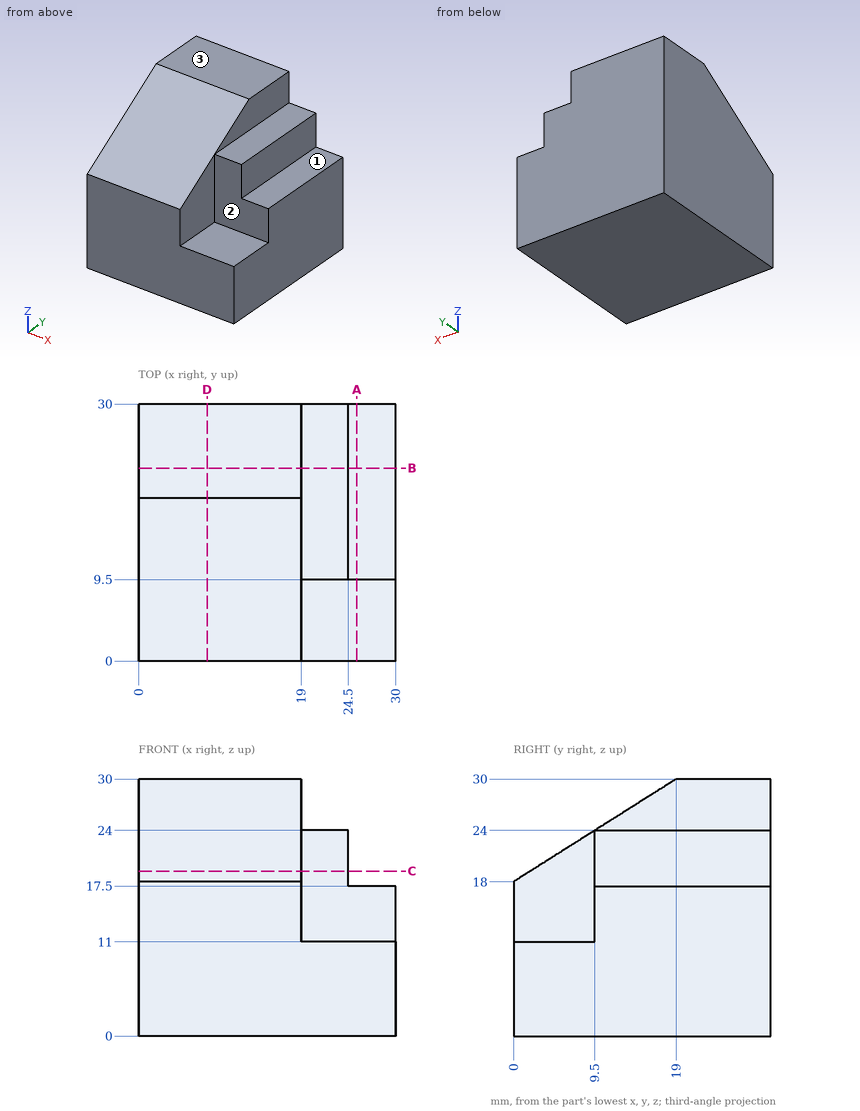
Drawing for the job (mm, zero at the part's lowest x, y, z). A direction names the side the tool comes from. Give positions to 0.01 mm unless a question says otherwise; leave off trailing zeros. Write each loop counter-clockwise with the first axis right and the second up, starting at its lowest first coordinate (ties: lowest second). Pieces come first, ordered by that corner, then holes. Notation, with made-up numbers: M 82,-23 L 93,-23 A22 ccw 93,-7 Z; hole C 37.25,-20.75 d1. An arc over 180 degrees is marked long. Return JSON: item names as keys, results as strings. Group by question number.
(1) Band-saw the part on C-C (z = 19.25). Give the cut face in (x, y), and give its area (3 significant figures).
(2) Flat gauge pins, fed straight in: pin 1 Ø1.5 at (x, y) = (21, 11.5) entering from -Z; pin 2 Ø1.6 at (x, y) = (22, 23.5) entering from +Z; pin 3 Ø5 at (y, z) = (19.5, 28) entering from +X; pin 4 Ø3 at (y, z) = (21, 20) entering from +X. Where does each tip first touch, or does it go through?
(3) Band-saw the part on B-B (y = 22.5). Give the cut face in (x, z).
(4) 3-axis set-ups, long thin cutter, end or side, ignore diameter. For the marked faces 1, 2 and 3: which of +Z, -Z, +X, -X, +Y, -Y reach the whole face in a straight line?
(5) Band-saw the part on D-D (x = 8). Give the cut face in (y, z).
(6) Drill centre lines: L1, parallel to Y at x = 20.5, z = 12; L2, parallel to X at y = 5.75, z = 15.5; L3, parallel to X at y = 25, z = 20.5. Where is each one in solid material? Low to high. Write a range as [from, to].
(7) Band-saw the part on A-A (x = 25.5). Give the cut face in (y, z), and give its area (3 significant figures).
Entries:
{
 "1": {"outline": "M 0,1.98 L 19,1.98 L 19,9.5 L 24.5,9.5 L 24.5,30 L 0,30 Z", "area": "645 mm^2"},
 "2": {"pin 1": "stops at z = 0", "pin 2": "stops at z = 24", "pin 3": "stops at x = 19", "pin 4": "stops at x = 24.5"},
 "3": {"outline": "M 0,0 L 30,0 L 30,17.5 L 24.5,17.5 L 24.5,24 L 19,24 L 19,30 L 0,30 Z"},
 "4": {"face 1": "+Z, +X, +Y, -Y", "face 2": "+Z, +X, -Y", "face 3": "+Z, +X, -X, +Y, -Y"},
 "5": {"outline": "M 0,0 L 30,0 L 30,30 L 19,30 L 0,18 Z"},
 "6": {"L1": "y = [9.5, 30]", "L2": "x = [0, 19]", "L3": "x = [0, 24.5]"},
 "7": {"outline": "M 0,0 L 30,0 L 30,17.5 L 9.5,17.5 L 9.5,11 L 0,11 Z", "area": "463 mm^2"}
}
